from build123d import *

# Parameters (mm, degrees)
SKETCH1_W           = 76.2
SKETCH1_H           = 76.2
SKETCH1_R           = 2.794
SKETCH1_R_2         = 33.02
BOSS_EXTRUDE1_DEPTH = 20.32
FILLET1_R           = 5.08
CUT_EXTRUDE1_DEPTH  = 88.58397342
CUT_EXTRUDE2_DEPTH  = 88.583973487


with BuildPart() as part:
    # Sketch1 → Boss-Extrude1 (new body)
    with BuildSketch(Plane(origin=(0, 0, 0), x_dir=(1, 0, 0), z_dir=(0, 1, 0))):
        Rectangle(SKETCH1_W, SKETCH1_H)
        with Locations(Location((33.02, 33.02, 0), (0, 0, 270))):
            Circle(SKETCH1_R, mode=Mode.SUBTRACT)
        with Locations(Location((33.02, -33.02, 0), (0, 0, 270))):
            Circle(SKETCH1_R, mode=Mode.SUBTRACT)
        with Locations(Location((-33.02, -33.02, 0), (0, 0, 270))):
            Circle(SKETCH1_R, mode=Mode.SUBTRACT)
        with Locations(Location((-33.02, 33.02, 0), (0, 0, 270))):
            Circle(SKETCH1_R, mode=Mode.SUBTRACT)
        with Locations(Location((0, 0, 0), (0, 0, 270))):
            Circle(SKETCH1_R_2, mode=Mode.SUBTRACT)
    extrude(amount=BOSS_EXTRUDE1_DEPTH)

    # Fillet1
    fillet1_edges = [part.edges().sort_by_distance(p)[0] for p in [
        (38.1, 10.16, 38.1),
        (-38.1, 10.16, 38.1),
        (-38.1, 10.16, -38.1),
        (38.1, 10.16, -38.1),
    ]]
    fillet(fillet1_edges, radius=FILLET1_R)

    # Sketch2 → Cut-Extrude1 (cut, through all)
    with BuildSketch(Plane.XY.offset(38.1)):
        with BuildLine():
            ThreePointArc((3.81, 10.16), (2.694076836, 12.854076836), (0, 13.97))
            Line((0, 13.97), (0, 6.35))
            ThreePointArc((0, 6.35), (2.694076836, 7.465923164), (3.81, 10.16))
        make_face()
        with BuildLine():
            Line((0, 6.35), (0, 13.97))
            ThreePointArc((0, 13.97), (-3.81, 10.16), (0, 6.35))
        make_face()
    extrude(amount=-CUT_EXTRUDE1_DEPTH, mode=Mode.SUBTRACT)

    # Sketch3 → Cut-Extrude2 (cut, through all)
    with BuildSketch(Plane(origin=(38.1, 0, 0), x_dir=(0, 0, -1), z_dir=(1, 0, 0))):
        with BuildLine():
            ThreePointArc((0, 13.97), (-3.81, 10.16), (0, 6.35))
            Line((0, 6.35), (0, 13.97))
        make_face()
        with BuildLine():
            Line((0, 13.97), (0, 6.35))
            ThreePointArc((0, 6.35), (2.694076836, 7.465923164), (3.81, 10.16))
            ThreePointArc((3.81, 10.16), (2.694076836, 12.854076836), (0, 13.97))
        make_face()
    extrude(amount=-CUT_EXTRUDE2_DEPTH, mode=Mode.SUBTRACT)


solid = part.part
For this review, take the finished solid that the model builds, in its own axes (mm). Round coordinates to 2 decimals unless told otherwise and drop trailing zeros. Order: outer loops, then holes, each group sorted by start corner. A loop starts at its lowest first (then second) coordinate and runs counter-clockwise, first axis right, second up. Notation, with made-up numbers: M 22,46 L 28,46 A35 ccw 28,79 Z; hole C -14.5,27.25 d1. An arc over 180 degrees is marked long. Use a Markdown table: item, result. Add a question column.
Item 1: Add section C-C, the plane z = -19. Give the boundary of the cut face in (x, y).
Item 2: Add section B-B, the plane x = -9. Give the boundary of the cut face in (y, z).
Item 3: Add section A-A, the plane y = 5.25. Give the boundary of the cut face in (x, z), then the cut area to 3 significant figures.
Item 4: To check wall thickness, follow line 1 along Z through (x, y) = (13.5, 4.5); line 2 along X through (y, z) = (18.25, 6.5); line 3 along X through (y, z) = (19.5, 4). State the ranges of each line that lie inside material, in increasing order.
Geometry results:
| question | item | result |
|---|---|---|
| 1 | outline | M -38.1,0 L -27.01,0 L -27.01,20.32 L -38.1,20.32 Z; M 27.01,0 L 38.1,0 L 38.1,20.32 L 27.01,20.32 Z |
| 2 | outline | M 0,-38.1 L 20.32,-38.1 L 20.32,-31.77 L 0,-31.77 Z; M 0,31.77 L 20.32,31.77 L 20.32,38.1 L 0,38.1 Z |
| 3 | outline | M -38.1,-33.02 A5.08 ccw -33.02,-38.1 L 33.02,-38.1 A5.08 ccw 38.1,-33.02 L 38.1,33.02 A5.08 ccw 33.02,38.1 L -33.02,38.1 A5.08 ccw -38.1,33.02 Z; hole C -33.02,-33.02 d5.59; hole C -33.02,33.02 d5.59; hole C 0,0 d66.04; hole C 33.02,-33.02 d5.59; hole C 33.02,33.02 d5.59 |
| 3 | area | 2,260 mm² |
| 4 | line 1 | z = -38.1 to -30.13, 30.13 to 38.1 |
| 4 | line 2 | x = -38.1 to -32.37, 32.37 to 38.1 |
| 4 | line 3 | x = -38.1 to -32.78, 32.78 to 38.1 |
